Geometry: final body of the model. Coordinates: model frame, mm. Face numbers are marked on the shaded views. A direction names the side the tool comes from. Round coordinates to 2 decimals unless told otherwise and drop trailing zeros. Loops run counter-clockwise (first coordinate to the right, second up) from the corner with the lowest first, then second, coordinate; pieces in that order, holes last. Notation, with made-up numbers: M 31,-24.5 L 37,-24.5 A25 ccw 37,5.5 Z; hole C -12,-12 d3. An arc over 180 degrees is marked long. Answer as a JSON object with one key per item and string values.
from build123d import *

# Parameters (mm, degrees)
SKETCH007_R           = 80
SKETCH007_R_2         = 55.15
EXTRUDE002_DEPTH      = 1
EXTRUDE_DEPTH         = 20
EXTRUDE003_DEPTH      = 2
EXTRUDE003_DEPTH_BACK = 10
SKETCH006_R           = 80
EXTRUDE001_DEPTH      = 2
CHAMFER_1_SIZE        = 1.5
CHAMFER_2_SIZE        = 1


with BuildPart() as extrude002:
    # Sketch007 → Extrude002 (new body)
    with BuildSketch(Plane.XY):
        Circle(SKETCH007_R)
        Circle(SKETCH007_R_2, mode=Mode.SUBTRACT)
    extrude(amount=-EXTRUDE002_DEPTH)


with BuildPart() as extrude002_1:
    # Extrude002 placement: moved
    add(extrude002.part.moved(Location((0, 0, 29.5))))


with BuildPart() as extrude_body:
    # Sketch005 → Extrude (new body, symmetric)
    with BuildSketch(Plane.XZ):
        with BuildLine():
            Line((-37.65, 3.8), (-26.65, 3.8))
            ThreePointArc((-26.65, 3.8), (-23.114466, 5.264466), (-21.65, 8.8))
            Line((-21.65, 8.8), (-21.65, 31.5))
            Line((-26.65, 31.5), (-21.65, 31.5))
            Line((-26.65, 31.5), (-26.65, 29.5))
            Line((-26.65, 29.5), (-23.65, 28.408089))
            Line((-23.65, 28.408089), (-23.65, 8.8))
            Line((-23.65, 8.8), (-26.65, 5.8))
            Line((-37.65, 5.8), (-26.65, 5.8))
            Line((-37.65, 5.8), (-40.65, 8.8))
            Line((-40.65, 8.8), (-40.65, 26.5))
            ThreePointArc((-40.65, 26.5), (-42.114466, 30.035534), (-45.65, 31.5))
            Line((-45.65, 29.5), (-45.65, 31.5))
            ThreePointArc((-42.65, 26.5), (-43.52868, 28.62132), (-45.65, 29.5))
            Line((-42.65, 11.8), (-42.65, 26.5))
            Line((-44.15, 11.8), (-42.65, 11.8))
            Line((-44.15, 11.8), (-42.65, 8.8))
            ThreePointArc((-42.65, 8.8), (-41.185534, 5.264466), (-37.65, 3.8))
        make_face()
    extrude(amount=EXTRUDE_DEPTH, both=True)


with BuildPart() as part_mirroring:
    # Part__Mirroring: instance of Extrude body
    add(extrude_body.part.mirror(Plane(origin=(0, 0, 0), x_dir=(0, -1, 0), z_dir=(1, 0, 0))))


with BuildPart() as frontplateoverhang:
    # Sketch008 → Extrude003 (new body, two sides)
    with BuildSketch(Plane.XY) as extrude003_sk:
        with BuildLine():
            ThreePointArc((41.88707, 27.027688), (0, 49.85), (-41.88707, 27.027688))
            Line((-41.88707, 27.027688), (-43.567594, 28.112048))
            ThreePointArc((43.567594, 28.112048), (0, 51.85), (-43.567594, 28.112048))
            Line((41.88707, 27.027688), (43.567594, 28.112048))
        make_face()
    extrude(amount=EXTRUDE003_DEPTH)
    extrude(extrude003_sk.sketch, amount=-EXTRUDE003_DEPTH_BACK)


with BuildPart() as frontplateoverhang_1:
    # Extrude003 placement: moved
    add(frontplateoverhang.part.moved(Location((0, 0, 29.5))))


with BuildPart() as part_mirroring001:
    # Part__Mirroring001: instance of frontplateoverhang
    add(frontplateoverhang_1.part.mirror(Plane(origin=(0, 0, 0), x_dir=(1, 0, 0), z_dir=(0, 1, 0))))


with BuildPart() as frontplate:
    # Sketch006 → Extrude001 (new body)
    with BuildSketch(Plane.XY):
        Circle(SKETCH006_R)
        with BuildLine():
            Line((-45.65, 0), (-45.65, 20))
            ThreePointArc((-46.938294, 22.027688), (-46.851168, 20.65994), (-45.65, 20))
            ThreePointArc((46.938287, 22.027703), (-8e-06, 51.85), (-46.938294, 22.027688))
            ThreePointArc((45.65, 20), (46.851173, 20.659947), (46.938287, 22.027703))
            Line((45.65, 0), (45.65, 20))
            Line((45.65, 0), (45.65, -20))
            ThreePointArc((46.938287, -22.027703), (46.851173, -20.659947), (45.65, -20))
            ThreePointArc((-46.938294, -22.027688), (-8e-06, -51.85), (46.938287, -22.027703))
            ThreePointArc((-45.65, -20), (-46.851168, -20.65994), (-46.938294, -22.027688))
            Line((-45.65, 0), (-45.65, -20))
        make_face(mode=Mode.SUBTRACT)
    extrude(amount=EXTRUDE001_DEPTH)


with BuildPart() as frontplate_1:
    # Extrude001 placement: moved
    add(frontplate.part.moved(Location((0, 0, 29.5))))

    # Fusion: union Extrude002, Part__Mirroring, Extrude body, Part__Mirroring001, frontplateoverhang
    add(extrude002_1.part)
    add(part_mirroring.part)
    add(extrude_body.part)
    add(part_mirroring001.part)
    add(frontplateoverhang_1.part)

    # Chamfer 1
    chamfer_1_edges = [frontplate_1.edges().sort_by_distance(p)[0] for p in [
        (-80, 0, 28.5),
        (0, 51.85, 19.5),
    ]]
    chamfer(chamfer_1_edges, length=CHAMFER_1_SIZE)

    # Chamfer 2
    chamfer_2_edges = [frontplate_1.edges().sort_by_distance(p)[0] for p in [
        (0, -51.85, 19.5),
    ]]
    chamfer(chamfer_2_edges, length=CHAMFER_2_SIZE)


solid = frontplate_1.part
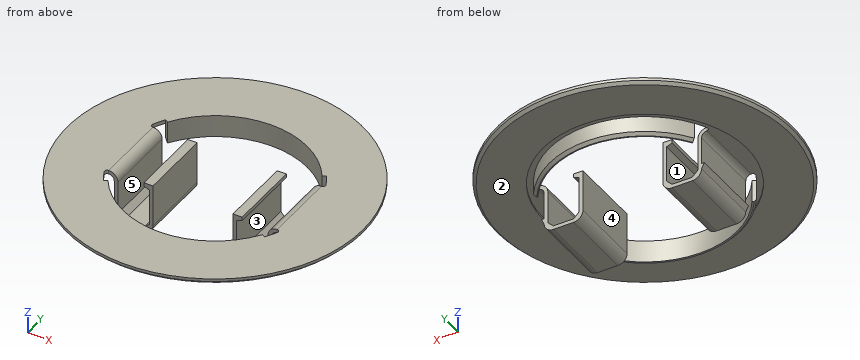
1) Pin query (flat end, axial travel): P1, Ø3, axis at x = -43, z = 14, coming from the +Y side; P2, Ø16, axis at y = 3.5, z = 18.5, coming from the +X side; P3, Ø12, axis at y = -26.5, z = 11.5, coming from the +X side; P4, Ø4.5, axis at y = 10, z = 20, coming from the -X side. Return the tip coordinate at first contact, or that it passes through.
Results:
{"P1": "y = 20", "P2": "x = 44.15", "P3": "through", "P4": "x = -42.65"}
2) Section query A-A (x = 0). Return the cut outline in (y, z), and give its area (3 significant figures).
Results:
{"outline": "M -80,30 L -78.5,28.5 L -55.15,28.5 L -55.15,29.5 L -51.85,29.5 L -51.85,20.5 L -50.85,19.5 L -49.85,19.5 L -49.85,31.5 L -80,31.5 Z; M 49.85,19.5 L 50.35,19.5 L 51.85,21 L 51.85,29.5 L 55.15,29.5 L 55.15,28.5 L 78.5,28.5 L 80,30 L 80,31.5 L 49.85,31.5 Z", "area": "206 mm2"}
3) Section query B-B (z = 15.75). Return the cut outline in (x, y), and give its area (3 significant figures).
Results:
{"outline": "M -42.65,-20 L -40.65,-20 L -40.65,20 L -42.65,20 Z; M -23.65,-20 L -21.65,-20 L -21.65,20 L -23.65,20 Z; M 21.65,-20 L 23.65,-20 L 23.65,20 L 21.65,20 Z; M 40.65,-20 L 42.65,-20 L 42.65,20 L 40.65,20 Z", "area": "320 mm2"}
4) Ray query, line 1 (X direction, y = -3.5, z = 23); line 2 (Y direction, x = 0, z = 28.9); line 3 (Y direction, x = 0, z = 29.1). Return the intervals inside material, ascending.
Results:
{"line 1": "-42.65 to -40.65, -23.65 to -21.65, 21.65 to 23.65, 40.65 to 42.65", "line 2": "-78.9 to -55.15, -51.85 to -49.85, 49.85 to 51.85, 55.15 to 78.9", "line 3": "-79.1 to -55.15, -51.85 to -49.85, 49.85 to 51.85, 55.15 to 79.1"}
5) Section query C-C (x = -33). Count the separate pieces of the cut face and the enclosed holes in it, and give its area (3 significant figures).
Results:
{"separate pieces": "3", "enclosed holes": "0", "area": "327 mm2"}
6) Pull-direction query (Y, two-part tool) for the marked faces 1 and 2; classes: +Y half, -Y half, draft (parallel to the pull), parting line (faces both ways), or undercut.
Results:
{"face 1": "undercut", "face 2": "draft"}
7) Reachability of the marked faces 3, 4 and 5 from +Z, -Z, +X, -X, +Y, -Y: full face, straight path, thin tool, end or side. Return the list, or none.
Results:
{"face 3": "none", "face 4": "+Z, -Z", "face 5": "+Z"}
